from build123d import *

# Parameters (mm, degrees)
SKETCH1_R           = 5
BOSS_EXTRUDE1_DEPTH = 3
SKETCH2_R           = 4.5
CUT_EXTRUDE1_DEPTH  = 2.5
SKETCH3_R           = 0.5
BOSS_EXTRUDE2_DEPTH = 15


with BuildPart() as part:
    # Sketch1 → Boss-Extrude1 (new body)
    with BuildSketch(Plane(origin=(0, 0, 0), x_dir=(1, 0, 0), z_dir=(0, 1, 0))):
        with Locations(Location((0, 0, 0), (0, 0, 270))):
            Circle(SKETCH1_R)
    extrude(amount=BOSS_EXTRUDE1_DEPTH)

    # Sketch2 → Cut-Extrude1 (cut)
    with BuildSketch(Plane(origin=(0, 3, 0), x_dir=(1, 0, 0), z_dir=(0, 1, 0))):
        with Locations(Location((0, 0, 0), (0, 0, 270))):
            Circle(SKETCH2_R)
    extrude(amount=-CUT_EXTRUDE1_DEPTH, mode=Mode.SUBTRACT)

    # Sketch3 → Boss-Extrude2 (add)
    with BuildSketch(Plane(origin=(0, 0.5, 0), x_dir=(1, 0, 0), z_dir=(0, 1, 0))):
        with Locations(Location((0, 0, 0), (0, 0, 270))):
            Circle(SKETCH3_R)
    extrude(amount=BOSS_EXTRUDE2_DEPTH)


solid = part.part
Design review of the part built by this model. Coordinates are the model's own, in mm. A direction names the side the tool comes from. Coordinates: 2 decimals unless noted, no trailing zeros. Order: outer loops, then holes, each group sorted by start corner. A loop starts at its lowest first (then second) coordinate and runs counter-clockwise, first axis right, second up. Notation, with made-up numbers: (53, 44.5) -> (96, 44.5) arc R7 cw to (96, 49.5) -> close; hole circle Ø5 at (-31.75, 51.25). An arc over 180 degrees is marked (long way). One line per item, written item: value.
1) Machinability: for faces 4 (the face through (0, 15.5, 0)), 5 (the face through (-1, 0.5, 0)), which of the approach directions +Z, -Z, +X, -X, +Y, -Y give a long, thin tool a straight path to every point of the face, cutting with its end or side? Answer none if there is none.
Output values:
face 4: +Z, -Z, +X, -X, +Y
face 5: +Y
2) To check wall thickness, follow probe 1 along X at (y, z) = (1.7, 0); probe 2 along Y at (x, z) = (0.75, 4.5); probe 3 along Y at (x, z) = (3, 2.5). State the ranges of each line that lie inside material, in increasing order. Write a range as [from, to].
Output values:
probe 1: x = [-5, -4.5], [-0.5, 0.5], [4.5, 5]
probe 2: y = [0, 3]
probe 3: y = [0, 0.5]
3) We need section A-A, the plane z = 0. Give the boundary of the cut face in (x, y), then the cut area to 3 significant figures.
Output values:
outline: (-5, 0) -> (5, 0) -> (5, 3) -> (4.5, 3) -> (4.5, 0.5) -> (0.5, 0.5) -> (0.5, 15.5) -> (-0.5, 15.5) -> (-0.5, 0.5) -> (-4.5, 0.5) -> (-4.5, 3) -> (-5, 3) -> close
area: 22.5 mm2
4) Clearance check with flat-ended pins moving along their axes: P1, Ø1.5, axis at x = -1.5, z = -3, coming from the -Y side; P2, Ø4, axis at y = 12, z = 0.5, coming from the +X side; P3, Ø1, axis at x = -1.5, y = 2.5, coming from the +Z side; P4, Ø1.5, axis at x = -2, z = -2, coming from the +Y side. State where each tip first meets the part, or that it passes through.
Output values:
P1: stops at y = 0
P2: stops at x = 0.5
P3: stops at z = 4.9
P4: stops at y = 0.5
5) We need section B-B, the plane y = 1. Give the boundary of the cut face in (x, z), then the cut area to 3 significant figures.
Output values:
outline: circle Ø10 at (0, 0); circle Ø1 at (0, 0); hole circle Ø9 at (0, 0)
area: 15.7 mm2
6) We need section D-D, the plane y = 9. Give the boundary of the cut face in (x, z), then the cut area to 3 significant figures.
Output values:
outline: circle Ø1 at (0, 0)
area: 0.785 mm2
7) We need section C-C, the plane x = 0. Give the boundary of the cut face in (y, z), then the cut area to 3 significant figures.
Output values:
outline: (0, -5) -> (3, -5) -> (3, -4.5) -> (0.5, -4.5) -> (0.5, -0.5) -> (15.5, -0.5) -> (15.5, 0.5) -> (0.5, 0.5) -> (0.5, 4.5) -> (3, 4.5) -> (3, 5) -> (0, 5) -> close
area: 22.5 mm2
8) Draft analysis for pull direction Z (two halves, no side actions). For faces 1 (the face through (-4.88, 1.48, -1.08)), 2 (the face through (1.352, 1.768, 4.292)), 3 (the face through (0, 0, 0)), state which applies: +Z half, -Z half, draft (parallel to the pull), parting line (faces both ways), or undercut.
Output values:
face 1: parting line
face 2: undercut
face 3: draft
